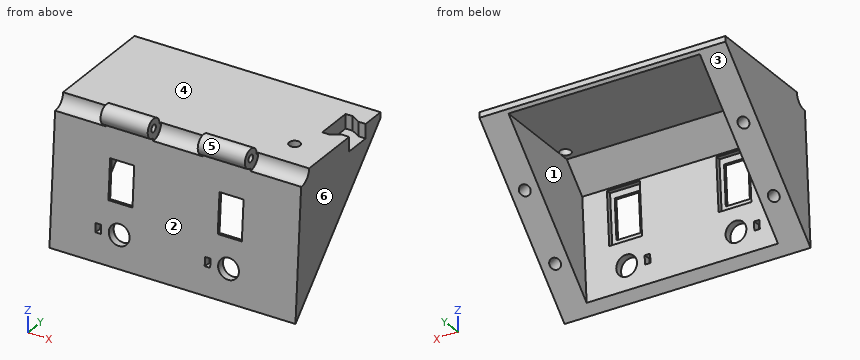
from build123d import *

# Parameters (mm, degrees)
PAD012_DEPTH    = 45
SKETCH023_R     = 3.45
PAD013_DEPTH    = 45
SKETCH024_W     = 18.6
SKETCH024_H     = 4.35
SKETCH024_W_2   = 18.3
SKETCH025_R     = 1.3
POCKET006_DEPTH = 45
POCKET007_DEPTH = 35
SKETCH027_R     = 2
POCKET008_DEPTH = 10
POCKET020_DEPTH = 5.2
SKETCH066_R     = 3.8
SKETCH066_W     = 8.8
SKETCH066_H     = 14.5
SKETCH066_W_2   = 2
SKETCH066_H_2   = 3.2
POCKET025_DEPTH = 3
SKETCH067_R     = 2
POCKET026_DEPTH = 13
SKETCH068_W     = 12
SKETCH068_H     = 19
POCKET027_DEPTH = 2


with BuildPart() as part:
    # Sketch022 → Pad012 (new body, symmetric)
    with BuildSketch(Plane.YZ):
        Polygon((0, 0), (-3.6088417733, -51.6088417733), (46, -2), (46, 0), align=None)
    extrude(amount=PAD012_DEPTH, both=True)

    # Sketch023 → Pad013 (join, symmetric)
    with BuildSketch(Plane.YZ):
        Circle(SKETCH023_R)
    extrude(amount=PAD013_DEPTH, both=True)

    # Sketch024 → Groove003 (revolve, cut)
    with BuildSketch(Plane.XZ):
        with Locations((-35.7, 2.175)):
            Rectangle(SKETCH024_W, SKETCH024_H)
        with Locations((0, 2.175)):
            Rectangle(SKETCH024_W_2, SKETCH024_H)
        with Locations((35.7, 2.175)):
            Rectangle(SKETCH024_W, SKETCH024_H)
    revolve(axis=Axis((0, 0, 0), (1, 0, 0)), mode=Mode.SUBTRACT)

    # Sketch025 → Pocket006 (cut, symmetric)
    with BuildSketch(Plane.YZ):
        Circle(SKETCH025_R)
    extrude(amount=POCKET006_DEPTH, both=True, mode=Mode.SUBTRACT)

    # Sketch026 → Pocket007 (cut, symmetric)
    with BuildSketch(Plane.YZ):
        Polygon((2, -12), (-1.4584733661, -61.4584733661), (57, -3), (11, -3), align=None)
    extrude(amount=POCKET007_DEPTH, both=True, mode=Mode.SUBTRACT)

    # Sketch027 (on Face5 of Pocket007) → Pocket008 (cut)
    with BuildSketch(Plane(origin=(0, 24, -24), x_dir=(0, 0.7071067812, 0.7071067812), z_dir=(0, 0.7071067812, -0.7071067812))):
        with Locations((5, 40)):
            Circle(SKETCH027_R)
        with Locations((-20, 40)):
            Circle(SKETCH027_R)
        with Locations((-20, -40)):
            Circle(SKETCH027_R)
        with Locations((5, -40)):
            Circle(SKETCH027_R)
    extrude(amount=-POCKET008_DEPTH, mode=Mode.SUBTRACT)

    # Sketch060 → Pocket020 (cut)
    with BuildSketch(Plane.XY):
        Polygon((45, 37.3), (42.4, 37.3), (39, 39.3), (36.4, 39.3), (36.4, 25.7), (39, 25.7), (42.4, 27.7), (45, 27.7), align=None)
    extrude(amount=-POCKET020_DEPTH, mode=Mode.SUBTRACT)

    # Sketch066 (on DatumPlane) → Pocket025 (cut)
    with BuildSketch(Plane(origin=(0, 0, 0), x_dir=(1, 0, 0), z_dir=(0, -0.9975640503, 0.0697564737))):
        with Locations((-20, -40)):
            Circle(SKETCH066_R)
        with Locations((20, -40)):
            Circle(SKETCH066_R)
        with Locations((-20, -22)):
            Rectangle(SKETCH066_W, SKETCH066_H)
        with Locations((20, -22)):
            Rectangle(SKETCH066_W, SKETCH066_H)
        with Locations((12.35, -40)):
            Rectangle(SKETCH066_W_2, SKETCH066_H_2)
        with Locations((-27.65, -40)):
            Rectangle(SKETCH066_W_2, SKETCH066_H_2)
    extrude(amount=-POCKET025_DEPTH, mode=Mode.SUBTRACT)

    # Sketch067 → Pocket026 (cut)
    with BuildSketch(Plane.XY):
        with Locations((33, 15)):
            Circle(SKETCH067_R)
    extrude(amount=-POCKET026_DEPTH, mode=Mode.SUBTRACT)

    # Sketch068 (on DatumPlane) → Pocket027 (cut)
    with BuildSketch(Plane(origin=(0, 2.9926921508, -0.2092694212), x_dir=(1, 0, 0), z_dir=(0, -0.9975640503, 0.0697564737))):
        with Locations((-20, -22)):
            Rectangle(SKETCH068_W, SKETCH068_H)
        with Locations((20, -22)):
            Rectangle(SKETCH068_W, SKETCH068_H)
    extrude(amount=POCKET027_DEPTH, mode=Mode.SUBTRACT)


solid = part.part
Can you work these out from the model? Positions are in its coordinate system, mm. Face numbers are marked on the shaded views. A direction names the side the tool comes from. Give positions to 0.01 mm unless a question says otherwise; leave off trailing zeros. Loops run counter-clockwise (first coordinate to the right, second up) from the corner with the lowest first, then second, coordinate; pieces in that order, holes last. Notation, with made-up numbers: (69.25, 57.5) - (117.25, 57.5) arc R21 cw to (117.25, 74.5) - close; hole circle Ø4 at (68.5, -11.5). An arc over 180 degrees is marked (long way). Answer as a JSON object with one key per item and string values.
Q1. Imagine slicing it at C-C on x = 33. Write out the boundary of the cut face in (y, z).
Geometry says:
{"outline": "(-3.61, -51.61) - (-0.56, -48.56) - (2, -12) - (11, -3) - (13, -3) - (13, 0) - (4.35, 0) arc R4.35 cw to (-0.3, -4.34) - close; (17, -3) - (45, -3) - (46, -2) - (46, 0) - (17, 0) - close"}
Q2. If we mould it in two halves opening along Z, with no side actions, what happens to the marked faces 4, 5 and 6? For each: pulls with the +Z half, pulls with the -Z half, needs draft (parallel to the pull), parting line crosses it, or undercut.
Geometry says:
{"face 4": "pulls with the +Z half", "face 5": "undercut", "face 6": "needs draft"}
Q3. Imagine slicing it at B-B on z = -24.5. Write out the boundary of the cut face in (x, y).
Geometry says:
{"outline": "(-45, -1.71) - (-24.4, -1.71) - (-24.4, -0.71) - (-26, -0.71) - (-26, 1.13) - (-35, 1.13) - (-35, 23.5) - (-45, 23.5) - close; (-15.6, -1.71) - (15.6, -1.71) - (15.6, -0.71) - (14, -0.71) - (14, 1.13) - (-14, 1.13) - (-14, -0.71) - (-15.6, -0.71) - close; (24.4, -1.71) - (45, -1.71) - (45, 23.5) - (35, 23.5) - (35, 1.13) - (26, 1.13) - (26, -0.71) - (24.4, -0.71) - close"}
Q4. Which directions (+Z, -Z, +X, -X, +Y, -Y) give clear straight access to the entire face, cutting with the end or side of a thin tool? Please do the marked faces 1, 2 and 3.
Geometry says:
{"face 1": "-Z, +Y", "face 2": "+X, -X, -Y", "face 3": "-Z, +X, -X, +Y"}
Q5. Imagine slicing it at D-D on x = 3.5. Write out the boundary of the cut face in (y, z), plus the area to 3 significant figures.
Geometry says:
{"outline": "(-3.61, -51.61) - (-0.56, -48.56) - (2, -12) - (11, -3) - (45, -3) - (46, -2) - (46, 0) - (4.35, 0) arc R4.35 cw to (-0.3, -4.34) - close", "area": "294 mm²"}
Q6. If I drill on L1, parallel to X at y = 16.5, z = -25.5; L2, parallel to Z at x = 12, y = 0; L3, parallel to Z at x = -17, y = 28, over which ranges is the centre line in solid material (lowest first)?
Geometry says:
{"L1": "-45 to -35, 35 to 45", "L2": "-38.49 to -1.3, 1.3 to 3.45", "L3": "-3 to 0"}
Q7. Imagine slicing it at A-A on x = -18. Write out the boundary of the cut face in (y, z), plus the area to 3 significant figures.
Geometry says:
{"outline": "(-3.61, -51.61) - (-0.56, -48.56) - (-0.19, -43.32) - (-3.02, -43.13) - close; (-2.56, -36.68) - (0.26, -36.88) - (0.63, -31.62) - (-1.2, -31.49) - (-1.04, -29.25) - (-2.04, -29.18) - close; (-1.03, -14.71) - (-0.03, -14.78) - (0.13, -12.54) - (1.95, -12.67) - (2, -12) - (11, -3) - (45, -3) - (46, -2) - (46, 0) - (3.45, 0) arc R3.45 ccw (long way) to (-0.24, -3.44) - close; hole circle Ø2.6 at (0, 0)", "area": "264 mm²"}
Q8. Will these pins go through, and if not, where does the flat tip stop? P1, Ø4, axis at y = 2.5, z = -1, coming from the +X side; P2, Ø1.3, axis at x = 43.5, z = -3, coming from the -Y side; P3, Ø5, axis at x = -9.5, z = -9.5, coming from the -Y side; P4, Ø2.5, axis at y = -1.5, z = 0, coming from the +X side.
Geometry says:
{"P1": "x = 45", "P2": "y = 2.37", "P3": "y = -0.84", "P4": "x = 26.4"}
